Design review of the part built by this model. Coordinates are the model's own, in mm. Face numbers are marked on the shaded views. Give positions to 0.01 mm unless a question says otherwise; leave off trailing zeros. Write each loop counter-clockwise with the first axis right and the second up, starting at its lowest first coordinate (ties: lowest second). Pieces come first, ordered by that corner, then holes. Notation, with made-up numbers: M -27.75,59 L 31.25,59 A16 cw 31.25,81 Z; hole C -10.5,46 d9. An arc over 180 degrees is marked long. Answer in a Markdown table with one row per item.
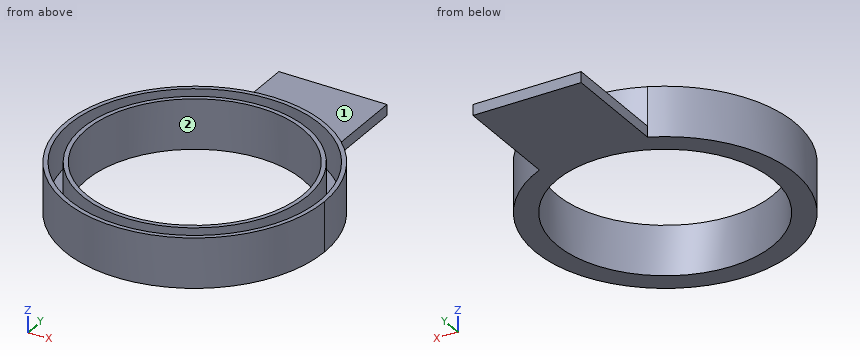
```python
from build123d import *

# Parameters (mm, degrees)
F0_R     = 50
F1_DEPTH = 5
F2_R     = 58
F2_R_2   = 52
F2_R_3   = 50
F3_DEPTH = 18


with BuildPart() as f1:
    # F0 (on Top) → F1 (new body)
    with BuildSketch(Plane.XY):
        with BuildLine():
            ThreePointArc((-25, 54.543561), (-32.403703, -50.497525), (60, 0))
            ThreePointArc((60, 0), (50.497525, 32.403703), (25, 54.543561))
            ThreePointArc((25, 54.543561), (0, 60), (-25, 54.543561))
        make_face()
        Circle(F0_R, mode=Mode.SUBTRACT)
        with BuildLine():
            ThreePointArc((-25, 54.543561), (0, 60), (25, 54.543561))
            Line((25, 54.543561), (25, 60))
            Line((25, 60), (25, 105))
            Line((25, 105), (-25, 105))
            Line((-25, 105), (-25, 54.543561))
        make_face()
    extrude(amount=F1_DEPTH)

    # F2 (on face) → F3 (join)
    with BuildSketch(Plane.XY.offset(5)):
        with BuildLine():
            ThreePointArc((-25, 54.543561), (-32.403703, -50.497525), (60, 0))
            ThreePointArc((60, 0), (50.497525, 32.403703), (25, 54.543561))
            ThreePointArc((25, 54.543561), (0, 60), (-25, 54.543561))
        make_face()
        Circle(F2_R, mode=Mode.SUBTRACT)
        Circle(F2_R_2)
        Circle(F2_R_3, mode=Mode.SUBTRACT)
    extrude(amount=F3_DEPTH)


solid = f1.part
```
1) The part is to be moulded in two halves that separate along Y. For the marked faces 1 and 2, say which applies: released by +Y, released by -Y, zero draft, split by the parting line, or undercut.
Geometry says:
| item | result |
|---|---|
| face 1 | zero draft |
| face 2 | undercut |
2) Add section D-D (x = -33.5). Write out the cut boundary in (y, z).
Geometry says:
| item | result |
|---|---|
| outline | M -49.78,0 L -37.12,0 L -37.12,23 L -39.77,23 L -39.77,5 L -47.35,5 L -47.35,23 L -49.78,23 Z; M 37.12,0 L 49.78,0 L 49.78,23 L 47.35,23 L 47.35,5 L 39.77,5 L 39.77,23 L 37.12,23 Z |
3) Add section A-A (x = 0). Write out the cut boundary in (y, z), and give its area (3 significant figures).
Geometry says:
| item | result |
|---|---|
| outline | M -60,0 L -50,0 L -50,23 L -52,23 L -52,5 L -58,5 L -58,23 L -60,23 Z; M 50,0 L 105,0 L 105,5 L 60,5 L 60,23 L 58,23 L 58,5 L 52,5 L 52,23 L 50,23 Z |
| area | 469 mm^2 |
4) Add section C-C (y = 11.5). Write out the cut boundary in (x, z).
Geometry says:
| item | result |
|---|---|
| outline | M -58.89,0 L -48.66,0 L -48.66,23 L -50.71,23 L -50.71,5 L -56.85,5 L -56.85,23 L -58.89,23 Z; M 48.66,0 L 58.89,0 L 58.89,23 L 56.85,23 L 56.85,5 L 50.71,5 L 50.71,23 L 48.66,23 Z |
5) Add section B-B (z = 17.25). Write out the cut boundary in (x, y), and give its area (3 significant figures).
Geometry says:
| item | result |
|---|---|
| outline | C 0,0 d104; M -25,54.54 A60 ccw long 60,0 A60 ccw 25,54.54 A60 ccw Z; hole C 0,0 d116; hole C 0,0 d100 |
| area | 1,380 mm^2 |
6) To check wall thickness, follow probe 1 along Y at (x, z) = (0, 12.75); probe 2 along Y at (x, z) = (42, 9.5); probe 3 along X at (y, z) = (-28, 20.5). State the ranges of each line that lie inside material, in increasing order. Write a range as [from, to].
Geometry says:
| item | result |
|---|---|
| probe 1 | [-60, -58], [-52, -50], [50, 52], [58, 60] |
| probe 2 | [-42.85, -40], [-30.66, -27.13], [27.13, 30.66], [40, 42.85] |
| probe 3 | [-53.07, -50.79], [-43.82, -41.42], [41.42, 43.82], [50.79, 53.07] |
7) Insertion check: P1, Ø8, axis at y = 53.5, z = 20.5, coming from the -X side; P2, Ø3, axis at x = -12.5, y = 59, coming from the +Z side; P3, Ø2.5, axis at y = 90, z = 1.5, coming from the +X side; P4, Ø15, axis at x = -12.5, y = 89, coming from the +Z side. Each pin has a flat end and moves straight along its axis. Give the tip position at first contact, or say it passes through.
Geometry says:
| item | result |
|---|---|
| P1 | x = -33.91 |
| P2 | z = 23 |
| P3 | x = 25 |
| P4 | z = 5 |
